Verification items for the finished model (mm, model axes). A direction names the side the tool comes from. Coordinates: 2 decimals unless noted, no trailing zeros. Order: outer loops, then holes, each group sorted by start corner. A loop starts at its lowest first (then second) coordinate and runs counter-clockwise, first axis right, second up. Notation, with made-up numbers: M 81,29 L 110,29 A8 ccw 110,35 Z; hole C 18,83 d2. An arc over 180 degrees is marked long. Use one line per item in the form item = value. Start each with the question number.
```python
from build123d import *

# Parameters (mm, degrees)
SKETCH_1_W          = 60
SKETCH_1_H          = 62
EXTRUDE_1_DEPTH     = 9
CUT_EXTRUDE_1_DEPTH = 20
SKETCH_3_R          = 5
EXTRUDE_2_DEPTH     = 4


with BuildPart() as part:
    # 草图1 → 凸台-拉伸1 (new body)
    with BuildSketch(Plane(origin=(0, 0, 0), x_dir=(1, 0, 0), z_dir=(0, 1, 0))):
        Rectangle(SKETCH_1_W, SKETCH_1_H)
    extrude(amount=EXTRUDE_1_DEPTH)

    # 草图2 → 切除-拉伸1 (cut)
    with BuildSketch(Plane.XZ):
        Polygon((6.215250205, 4), (25.8, 4), (28.7, 15.937822174), (23.906181585, 25.383019067), (25.236860279, 27.687822174), (30, 24.937822174), (30, 31), (-30, 31), (-30, -31), (30, -31), (30, -24.937822174), (25.236860279, -27.687822174), (23.906181585, -25.383019067), (28.7, -15.937822174), (25.8, -4), (6.215250205, -4), (3.715250205, -7.102951113), (2.215250205, -7.102951113), (2.215250205, 0), (2.215250205, 7.102951113), (3.715250205, 7.102951113), align=None)
    extrude(amount=-CUT_EXTRUDE_1_DEPTH, mode=Mode.SUBTRACT)

    # 草图3 → 凸台-拉伸2 (add)
    with BuildSketch(Plane(origin=(0, 9, 0), x_dir=(1, 0, 0), z_dir=(0, 1, 0))):
        Polygon((2.215250205, 0), (30, 0), (30, 24.937822174), (25.236860279, 27.687822174), (23.906181585, 25.383019067), (28.7, 15.937822174), (25.8, 4), (6.215250205, 4), (3.715250205, 7.102951113), (2.215250205, 7.102951113), align=None)
        with BuildLine():
            Line((23.906181585, 25.383019067), (25.236860279, 27.687822174))
            Line((25.236860279, 27.687822174), (16.955072532, 32.35575698))
            ThreePointArc((16.955072532, 32.35575698), (18.817138095, 30.522363707), (19.5, 28))
            ThreePointArc((19.5, 28), (12.029027225, 23.65324333), (11.942282582, 32.296286956))
            Line((11.942282582, 32.296286956), (2.215250205, 26.50547261))
            Line((2.215250205, 26.50547261), (2.215250205, 7.102951113))
            Line((2.215250205, 7.102951113), (3.715250205, 7.102951113))
            Line((3.715250205, 7.102951113), (6.215250205, 4))
            Line((6.215250205, 4), (25.8, 4))
            Line((25.8, 4), (28.7, 15.937822174))
            Line((28.7, 15.937822174), (23.906181585, 25.383019067))
        make_face()
        with Locations((14.5, 28)):
            Circle(SKETCH_3_R)
        Polygon((25.236860279, -27.687822174), (30, -24.937822174), (30, 0), (2.215250205, 0), (2.215250205, -7.102951113), (3.715250205, -7.102951113), (6.215250205, -4), (25.8, -4), (28.7, -15.937822174), (23.906181585, -25.383019067), align=None)
        with BuildLine():
            Line((16.955072532, -32.35575698), (25.236860279, -27.687822174))
            Line((25.236860279, -27.687822174), (23.906181585, -25.383019067))
            Line((23.906181585, -25.383019067), (28.7, -15.937822174))
            Line((28.7, -15.937822174), (25.8, -4))
            Line((25.8, -4), (6.215250205, -4))
            Line((6.215250205, -4), (3.715250205, -7.102951113))
            Line((3.715250205, -7.102951113), (2.215250205, -7.102951113))
            Line((2.215250205, -7.102951113), (2.215250205, -26.50547261))
            Line((2.215250205, -26.50547261), (11.942282582, -32.296286956))
            ThreePointArc((11.942282582, -32.296286956), (12.029027225, -23.65324333), (19.5, -28))
            ThreePointArc((19.5, -28), (18.817138095, -30.522363707), (16.955072532, -32.35575698))
        make_face()
        with Locations((14.5, -28)):
            Circle(SKETCH_3_R)
    extrude(amount=EXTRUDE_2_DEPTH)


solid = part.part
```
1. Tool access check on faces 1 (the flat face through (4.95, 4.44, 5.57)), 2 (the flat face through (26.34, 4.44, 20.59)), 3 (the flat face through (3, 4, 7.103)), 4 (the flat face through (3, 4, -7.103)). Record the directions out of +Z, -Z, +X, -X, +Y, -Y that give a thin tool (end or side, any length) a straight path to the whole face; none if there is none.
2. Cross-section at A-A on y = 1. Enter the section's corners in (x, z).
3. Cross-section at C-C on y = 10.25. Enter the section's corners in (x, z), and give its area (3 significant figures).
4. Depth check by flat-ended pin: P1, Ø6, axis at x = 12, z = 25.5, coming from the -Y side; P2, Ø2.5, axis at x = 17.5, y = 2.5, coming from the -Z side; P3, Ø1.7, axis at x = 3, y = 3, coming from the +Z side; P4, Ø3, axis at y = 8.5, z = 19.5, coming from the -X side. Enter the tip coordinate at first touch or a pass-through.
5. Release check for a two-part mould opening along Z. For faces 5 (the flat face through (20, 0, 0)), 6 (the flat face through (27.23, 4.44, 9.89)), 7 (the flat face through (27.652, 6.409, -26.294)) record: pulls with the +Z half, pulls with the -Z half, needs draft (parallel to the pull), parting line crosses it, or undercut.
6. Cross-section at B-B on x = 13.25. Enter the section's corners in (y, z).
7. Cross-section at D-D on x = 18.75. Enter the section's corners in (y, z).
8. Material ranges on line 1 along Y through (x, z) = (14.75, 14.5); line 2 along Z through (x, y) = (20.5, 7.75); line 3 along Z through (x, y) = (3.5, 3.75), recorded low to high.
Final values:
q1.face_1 = +Z, -Y
q1.face_2 = -X, -Y
q1.face_3 = +Z, -X, -Y
q1.face_4 = -Z, -X, -Y
q2.outline = M 2.22,-7.1 L 3.72,-7.1 L 6.22,-4 L 25.8,-4 L 28.7,-15.94 L 23.91,-25.38 L 25.24,-27.69 L 30,-24.94 L 30,24.94 L 25.24,27.69 L 23.91,25.38 L 28.7,15.94 L 25.8,4 L 6.22,4 L 3.72,7.1 L 2.22,7.1 Z
q3.outline = M 2.22,-26.51 L 11.94,-32.3 A5 ccw 16.96,-32.36 L 25.24,-27.69 L 30,-24.94 L 30,24.94 L 25.24,27.69 L 16.96,32.36 A5 ccw 11.94,32.3 L 2.22,26.51 Z
q3.area = 1,650 mm2
q4.P1 = 9
q4.P2 = -4
q4.P3 = 7.1
q4.P4 = 2.22
q5.face_5 = needs draft
q5.face_6 = undercut
q5.face_7 = pulls with the -Z half
q6.outline = M 0,-4 L 9,-4 L 9,-32.84 L 13,-32.84 L 13,32.84 L 9,32.84 L 9,4 L 0,4 Z
q7.outline = M 0,-4 L 9,-4 L 9,-31.34 L 13,-31.34 L 13,31.34 L 9,31.34 L 9,4 L 0,4 Z
q8.line_1 = 9 to 13
q8.line_2 = -4 to 4
q8.line_3 = -7.1 to 7.1
